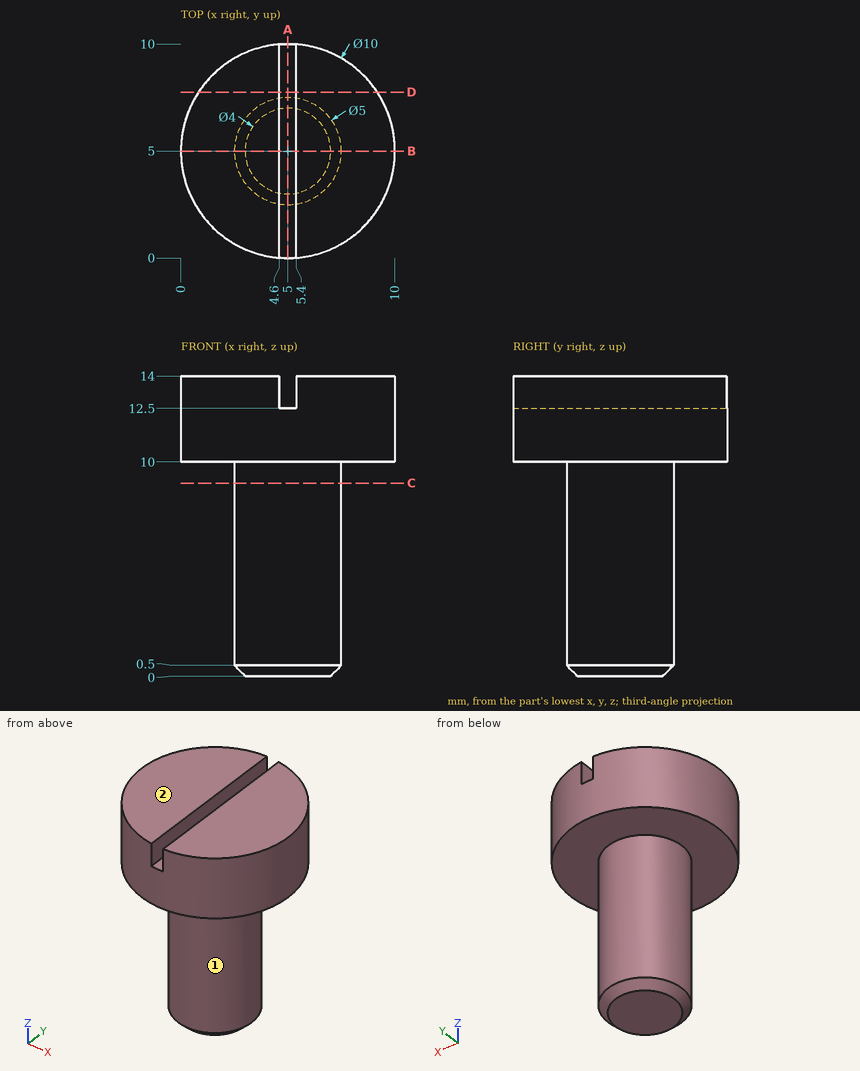
Answer from the drawing. Dimensions are ordinates in mm from the lowest x, y and z of the part. A direction names the side the tool comes from. Give positions to 0.01 mm unless a question says otherwise; leave off trailing zeros. Write each loop counter-clockwise with the first axis right and the second up, starting at its lowest first coordinate (ties: lowest second). Pieces come first, ordered by that corner, then holes. Notation, with made-up numbers: (-39, 34.5) -> (-18, 34.5) arc R31 ccw to (-18, 63.5) -> close; hole circle Ø5 at (-24, 70.25). An arc over 180 degrees is marked (long way). Use a Markdown table: item, result.
(1) Section D-D, the plane y = 7.75 is taken. Determine the outline of the cut face in (x, z).
Return value:
| item | result |
|---|---|
| outline | (0.82, 10) -> (9.18, 10) -> (9.18, 14) -> (5.4, 14) -> (5.4, 12.5) -> (4.6, 12.5) -> (4.6, 14) -> (0.82, 14) -> close |
(2) Section B-B, the plane y = 5 is taken. Determine the outline of the cut face in (x, z), then the cut area to 4 significant figures.
Return value:
| item | result |
|---|---|
| outline | (0, 10) -> (2.5, 10) -> (2.5, 0.5) -> (3, 0) -> (7, 0) -> (7.5, 0.5) -> (7.5, 10) -> (10, 10) -> (10, 14) -> (5.4, 14) -> (5.4, 12.5) -> (4.6, 12.5) -> (4.6, 14) -> (0, 14) -> close |
| area | 88.55 mm2 |
(3) Section A-A, the plane x = 5 is taken. Determine the outline of the cut face in (y, z), then the cut area to 4 significant figures.
Return value:
| item | result |
|---|---|
| outline | (0, 10) -> (2.5, 10) -> (2.5, 0.5) -> (3, 0) -> (7, 0) -> (7.5, 0.5) -> (7.5, 10) -> (10, 10) -> (10, 12.5) -> (0, 12.5) -> close |
| area | 74.75 mm2 |
(4) Section C-C, the plane z = 9 is taken. Determine the outline of the cut face in (x, y).
Return value:
| item | result |
|---|---|
| outline | circle Ø5 at (5, 5) |
(5) For the marked faces 1 and 2, determine the directions among +Z, -Z, +X, -X, +Y, -Y from which every point of the face is accessible in a straight line to the end or side of a thin tool.
Return value:
| item | result |
|---|---|
| face 1 | -Z |
| face 2 | +Z, +X, -X, +Y, -Y |
(6) Find the intervals of material crossed by probe 1 along Z at (x, y) = (7.5, 8); probe 2 along Z at (x, y) = (5, 0.75); probe 3 along Y at (x, z) = (6.5, 4.25), in increasing order. Write a range as from..to.
Return value:
| item | result |
|---|---|
| probe 1 | 10..14 |
| probe 2 | 10..12.5 |
| probe 3 | 3..7 |
(7) Flat-ended cylindrical pins translate along their axes: P1, Ø1.6, axis at y = 6, z = 13.5, coming from the +X side; P2, Ø6, axis at x = 6, z = 8.5, coming from the -Y side; P3, Ø1.2, axis at y = 3.5, z = 13, coming from the -X side; P4, Ø2, axis at x = 8, y = 8.5, coming from the -Z side. Find the tip coordinate at first contact, or state that the pin passes through.
Return value:
| item | result |
|---|---|
| P1 | x = 10 |
| P2 | y = 0 |
| P3 | x = 0.08 |
| P4 | z = 10 |
